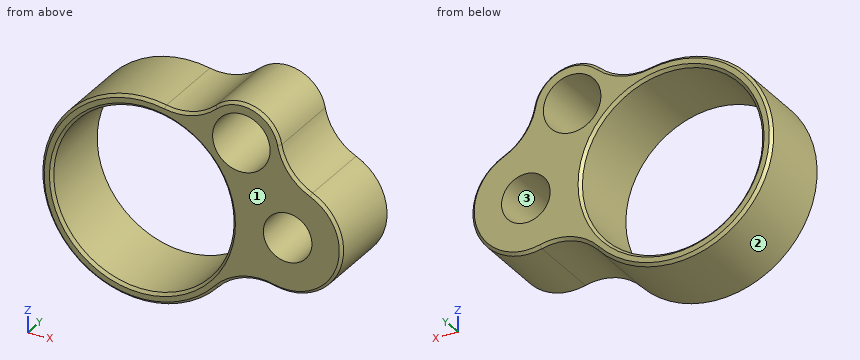
```python
from build123d import *

# Parameters (mm, degrees)
F0_R     = 16.15
F0_R_2   = 4.35
F0_R_3   = 5.15
F1_DEPTH = 15
F2_R     = 10
F3_SIZE  = 0.5


with BuildPart() as f1:
    # F0 (on Front) → F1 (new body)
    with BuildSketch(Plane.XZ):
        with BuildLine():
            ThreePointArc((17.472067, -4.726189), (35.382893, -2.650248), (21.204868, 8.489359))
            ThreePointArc((21.204868, 8.489359), (21.28794, 20.805684), (10.613035, 14.661974))
            ThreePointArc((10.613035, 14.661974), (-17.063659, -6.036683), (17.472067, -4.726189))
        make_face()
        Circle(F0_R, mode=Mode.SUBTRACT)
        with Locations((26, 0)):
            Circle(F0_R_2, mode=Mode.SUBTRACT)
        with Locations((17.713029, 14.671353)):
            Circle(F0_R_3, mode=Mode.SUBTRACT)
    extrude(amount=-F1_DEPTH)

    # F2
    f2_edges = [f1.edges().sort_by_distance(p)[0] for p in [
        (10.613035, 7.5, 14.661974),
        (21.204868, 7.5, 8.489359),
        (17.472067, 7.5, -4.726189),
    ]]
    fillet(f2_edges, radius=F2_R)

    # F3
    f3_edges = [f1.edges().sort_by_distance(p)[0] for p in [
        (-17.286785, 0, -5.364427),
        (-17.286785, 15, -5.364427),
        (-16.15, 15, 0),
        (-16.15, 0, 0),
    ]]
    chamfer(f3_edges, length=F3_SIZE)


solid = f1.part
```
Check sheet for the modelled part. Datum: model origin and axes. Units: mm. Face numbers are marked on the shaded views. Round coordinates to 2 decimals unless told otherwise and drop trailing zeros. Loops run counter-clockwise (first coordinate to the right, second up) from the corner with the lowest first, then second, coordinate; pieces in that order, holes last. Notation, with made-up numbers: (21.25, -12.75) -> (72.25, -12.75) arc R19 cw to (72.25, 12.25) -> close; hole circle Ø7 at (21.5, 32). An arc over 180 degrees is marked (long way). Answer in a Markdown table with one row per item.
Q1. Sectioned sample at C-C on y = 4. Give the number of separate pieces and of enclosed holes in the cut face, then the cut area to 3 significant figures.
Data:
| item | result |
|---|---|
| separate pieces | 1 |
| enclosed holes | 3 |
| area | 540 mm^2 |
Q2. Release check for a two-part mould opening along Z. For the marked faces 1, 2 and 3 record: released by +Z, released by -Z, zero draft, split by the parting line, or undercut.
Data:
| item | result |
|---|---|
| face 1 | zero draft |
| face 2 | split by the parting line |
| face 3 | undercut |
Q3. Thickness scan on L1, parallel to X at y = 8.25, z = 14.5; L2, parallel to X at y = 12, z = 14; L3, parallel to Z at x = 0, y = 9.5. Record the ranges inside material, lowest first.
Data:
| item | result |
|---|---|
| L1 | x = -10.83 to -7.11, 7.11 to 12.57, 22.86 to 25.09 |
| L2 | x = -11.47 to -8.05, 8.05 to 12.61, 22.82 to 25.28 |
| L3 | z = -18.1 to -16.15, 16.15 to 18.1 |
Q4. Go/stop test with flat-tipped pins: P1, Ø6, axis at y = 10.5, z = 4.5, coming from the -X side; P2, Ø1, axis at x = -5, y = 3.5, coming from the -Z side; P3, Ø2, axis at x = -10.5, y = 13.5, coming from the +Z side; P4, Ø7, axis at x = 26, z = 0, coming from the +Y side. Record where each tip stops, or that it passes through.
Data:
| item | result |
|---|---|
| P1 | stops at x = -18.04 |
| P2 | stops at z = -17.53 |
| P3 | stops at z = 15.41 |
| P4 | passes through |
Q5. Sectioned sample at A-A on z = 0. Enter the section's corners in (x, y).
Data:
| item | result |
|---|---|
| outline | (-18.1, 0.5) -> (-17.6, 0) -> (-16.65, 0) -> (-16.15, 0.5) -> (-16.15, 14.5) -> (-16.65, 15) -> (-17.6, 15) -> (-18.1, 14.5) -> close; (16.15, 0.5) -> (16.65, 0) -> (21.65, 0) -> (21.65, 15) -> (16.65, 15) -> (16.15, 14.5) -> close; (30.35, 0) -> (35.25, 0) -> (35.75, 0.5) -> (35.75, 14.5) -> (35.25, 15) -> (30.35, 15) -> close |
Q6. Sectioned sample at B-B on x = 0. Enter the section's corners in (y, z), then the cut area to 3 significant figures.
Data:
| item | result |
|---|---|
| outline | (0, -17.6) -> (0.5, -18.1) -> (14.5, -18.1) -> (15, -17.6) -> (15, -16.65) -> (14.5, -16.15) -> (0.5, -16.15) -> (0, -16.65) -> close; (0, 16.65) -> (0.5, 16.15) -> (14.5, 16.15) -> (15, 16.65) -> (15, 17.6) -> (14.5, 18.1) -> (0.5, 18.1) -> (0, 17.6) -> close |
| area | 57.5 mm^2 |
